```python
from build123d import *

# Parameters (mm, degrees)
SKETCH2_R           = 22
SKETCH2_R_2         = 2.75
BOSS_EXTRUDE1_DEPTH = 2.4
SKETCH3_R           = 3.9
BOSS_EXTRUDE2_DEPTH = 9
SKETCH4_R           = 11
BOSS_EXTRUDE3_DEPTH = 28


with BuildPart() as part:
    # Sketch2 → Boss-Extrude1 (new body)
    with BuildSketch(Plane(origin=(0, 0, 0), x_dir=(1, 0, 0), z_dir=(0, 1, 0))):
        Circle(SKETCH2_R)
        with Locations((15.155444566, 8.75)):
            Circle(SKETCH2_R_2, mode=Mode.SUBTRACT)
        with Locations((-15.155444566, 8.75)):
            Circle(SKETCH2_R_2, mode=Mode.SUBTRACT)
        with Locations((0, -17.5)):
            Circle(SKETCH2_R_2, mode=Mode.SUBTRACT)
    extrude(amount=BOSS_EXTRUDE1_DEPTH)

    # Sketch3 → Boss-Extrude2 (add)
    with BuildSketch(Plane(origin=(0, 2.4, 0), x_dir=(1, 0, 0), z_dir=(0, 1, 0))):
        Circle(SKETCH3_R)
    extrude(amount=BOSS_EXTRUDE2_DEPTH)

    # Sketch4 → Boss-Extrude3 (add)
    with BuildSketch(Plane.XZ):
        Circle(SKETCH4_R)
    extrude(amount=BOSS_EXTRUDE3_DEPTH)


solid = part.part
```
Input: part model. Units: mm. Frame: model coordinates. A direction names the side the tool comes from. Give positions to 0.01 mm unless a question says otherwise; leave off trailing zeros. Order: outer loops, then holes, each group sorted by start corner. A loop starts at its lowest first (then second) coordinate and runs counter-clockwise, first axis right, second up. Notation, with made-up numbers: M 7.5,69.25 L 64.5,69.25 A29 cw 64.5,108.25 Z; hole C 33.5,-21 d4. An arc over 180 degrees is marked long. Return JSON: item names as keys, results as strings.
Item 1: Access query for faces 4 (the cylindrical face through (-2.38, -13.8, -10.74)), 5 (the cylindrical face through (-2.87, 6.84, -2.64)), 6 (the flat face through (0, -28, 0)). Directions: +Z, -Z, +X, -X, +Y, -Y. A direction counts if a zero-diameter tool reaches every point of the face in a straight line with its end or side. Return the directions, or none.
Solutions:
{"face 4": "-Y", "face 5": "+Y", "face 6": "+Z, -Z, +X, -X, -Y"}
Item 2: Pull-direction query (X, two-part tool) for faces 1 (the cylindrical face through (-4.769, 1.183, 21.477)), 2 (the flat face through (5, 0, -10)), 3 (the cylindrical face through (17.778, 1.183, -9.576)); classes: +X half, -X half, draft (parallel to the pull), parting line (faces both ways), or undercut.
Solutions:
{"face 1": "parting line", "face 2": "draft", "face 3": "undercut"}
Item 3: Cut plane C-C (z = 17.5). Return loops of the section in (x, y), then the cut area to 3 significant figures.
Solutions:
{"outline": "M -13.33,0 L -2.75,0 L -2.75,2.4 L -13.33,2.4 Z; M 2.75,0 L 13.33,0 L 13.33,2.4 L 2.75,2.4 Z", "area": "50.8 mm^2"}
Item 4: Cut plane A-A (x = 0). Return loops of the section in (y, z), then the cut area to 3 significant figures.
Solutions:
{"outline": "M -28,-11 L 0,-11 L 0,-22 L 2.4,-22 L 2.4,-3.9 L 11.4,-3.9 L 11.4,3.9 L 2.4,3.9 L 2.4,14.75 L 0,14.75 L 0,11 L -28,11 Z; M 0,20.25 L 2.4,20.25 L 2.4,22 L 0,22 Z", "area": "779 mm^2"}
Item 5: Cut plane D-D (z = 0). Return loops of the section in (x, y).
Solutions:
{"outline": "M -22,0 L -11,0 L -11,-28 L 11,-28 L 11,0 L 22,0 L 22,2.4 L 3.9,2.4 L 3.9,11.4 L -3.9,11.4 L -3.9,2.4 L -22,2.4 Z"}
Item 6: Cut plane B-B (z = -10). Return loops of the section in (x, y), then the cut area to 3 significant figures.
Solutions:
{"outline": "M -19.6,0 L -17.6,0 L -17.6,2.4 L -19.6,2.4 Z; M -12.71,0 L -4.58,0 L -4.58,-28 L 4.58,-28 L 4.58,0 L 12.71,0 L 12.71,2.4 L -12.71,2.4 Z; M 17.6,0 L 19.6,0 L 19.6,2.4 L 17.6,2.4 Z", "area": "327 mm^2"}
Item 7: Ray query, probe 1 along Z at (x, y) = (0, 0.6); probe 2 along X at (y, z) = (0.9, -8.75); probe 3 along Y at (x, z) = (-10, -10). Return the intervals inside material, ascending.
Solutions:
{"probe 1": "-22 to 14.75, 20.25 to 22", "probe 2": "-20.19 to -17.91, -12.41 to 12.41, 17.91 to 20.19", "probe 3": "0 to 2.4"}
Item 8: First-contact query: P1, Ø3, axis at x = -5, z = -16.5, coming from the -Y side; P2, Ø3, axis at x = 1, z = 16.5, coming from the +Y side; P3, Ø4.5, axis at x = 0, z = 17.5, coming from the -Y side; P4, Ø12, axis at x = 8.5, y = -11, coming from the -Z side. Flat tips, straight axial feed; report the tip coordinate or a pass-through.
Solutions:
{"P1": "y = 0", "P2": "y = 2.4", "P3": "through", "P4": "z = -10.71"}
